Read the model definition and answer for the solid it produces. Units are mm, in the model's axes. Face numbers are marked on the shaded views. A direction names the side the tool comes from. Give positions to 0.01 mm unless a question says otherwise; leave off trailing zeros. Write each loop counter-clockwise with the first axis right and the second up, starting at its lowest first coordinate (ties: lowest second). Pieces come first, ordered by that corner, then holes. Notation, with made-up numbers: M 35.25,58 L 78.25,58 A11 cw 78.25,63 Z; hole C 68.5,-32 d7. An arc over 180 degrees is marked long. Answer as CSV lines item,"result". Start each with the question number.
Autodesk Inventor part; units mm, degrees
ref_plane "Work Plane1" through (29, 0, 0) normal (0, -1, 0) x (1, 0, 0)
ref_plane "YZ Plane" through (0, 0, 0) normal (1, 0, 0) x (0, 1, 0)
ref_plane "XZ Plane" through (0, 0, 0) normal (0, 1, 0) x (-1, 0, 0)
sketch "Sketch1" plane through (0, 0, 0) normal (0, 0, 1) x (1, 0, 0)
  line L0 (-1.1667, 0) -> (35, 0)
  line L1 (35, 0) -> (35, 2.5)
  line L2 (35, 2.5) -> (19, 2.5)
  line L3 (19, 2.5) -> (18.5091, 2.5)
  line L4 (18.5091, 2.5) -> (0, 2.5)
  line L5 (0, 2.5) -> (0, 4.25)
  line L6 (0, 4.25) -> (-5, 4.25)
  line L7 (-5, 4.25) -> (-5, 2.3094)
  line L8 (-5, 2.3094) -> (-2.5, 2.3094)
  line L9 (-2.5, 2.3094) -> (-1.1667, 0)
  line L10 (-13, 0) -> (43, 0)
  line L11 (0, -0.85) -> (0, 5.1)
  line L12 (19, 2.5) -> (0, 2.5) construction
  dimension "d1" = 16
  dimension "d2" = 0.4909
  dimension "d3" = 5
  dimension "d4" = 2.5
  dimension "d5" = 60
  dimension "d6" = 5
  dimension "d7" = 5
  dimension "d8" = 4.6188
  dimension "d9" = 8.5
  dimension "d26" = 35
revolve "Body" add sketch "Sketch1" angle 360 about axis through (-1.1667, 0, 0) along (1, 0, 0)
sketch "Sketch2" plane through (-5, 0, 0) normal (-1, 0, 0) x (0, 0, 1)
  circle A0 centre (0, 0) radius 2.3094
  line L0 (0, -5.95) -> (0, 5.95)
  line L1 (-5.95, 0) -> (5.95, 0)
  line L2 (2.3094, 0) -> (1.1547, -2)
  line L3 (1.1547, -2) -> (-1.1547, -2)
  line L4 (-1.1547, -2) -> (-2.3094, 0)
  line L5 (-2.3094, 0) -> (-1.1547, 2)
  line L6 (-1.1547, 2) -> (1.1547, 2)
  line L7 (1.1547, 2) -> (2.3094, 0)
extrude "Slot" add sketch "Sketch2" against normal up to next contours L7 A0 | A0 L2 | L6 L0 A0 | A0 L0 L3 | L0 L6 A0 | A0 L3 L0 | L4 A0 | A0 L5
fillet "Fillet1" radius 0.5 1 edges at (-5, -4.25, 0)
thread "Thread"
chamfer "Chamfer1" distance 0.4908 distance2 0.4908 1 edges at (35, -2.5, 0) measured on face at (35, -0.7192, 0.1653)
ref_plane "Work Plane1" through (29, 0, 0) normal (0, -1, 0) x (1, 0, 0)
fillet "Fillet2" radius 0.1 1 edges at (0, -2.5, 0)
equation "\"d1\" = GEL"
equation "\"d3\" = KOH"
equation "\"d4\" = INTI"
equation "\"d6\" = GD"
equation "\"d7\" = BDM"
equation "\"d8\" = 1.1547 * SW"
equation "\"d9\" = KOD"
equation "\"d17\" = RR"
equation "\"d13\" = GEL"
equation "\"d15\" = -0.5 * SPD + 0.5 * GD"
equation "\"d16\" = GUL"
equation "\"d30\" = R"
equation "\"GD\" = NND"
equation "\"GEL\" = 16"
equation "\"KOD\" = 8.5"
equation "\"KOH\" = NND"
equation "\"INTI\" = 2.5"
equation "\"GAL\" = 0.61345 * PTC"
equation "\"GUL\" = 0.61345 * PTC"
equation "\"BDM\" = NND"
equation "\"SW\" = 4"
equation "\"RR\" = 0.1 * NND"
equation "\"SPD\" = NND - 1.2269 * PTC"
equation "\"R\" = 0.1"
equation "\"PHH\" = 0.13"
equation "\"GD1\" = THREADDIA - 1.2269 * PTC"
equation "\"THREADDIA\" = 5"
equation "\"FAWI\" = 45deg"
equation "\"PTC\" = 0.8"
equation "\"KOH1\" = 4.5"
equation "\"NND\" = 5"
equation "\"TOA\" = 30deg"
equation "\"E0\" = 1.155 * SW"
properties part number "AS 1420 - 1973 - M5 x 20" material "Steel, Mild"
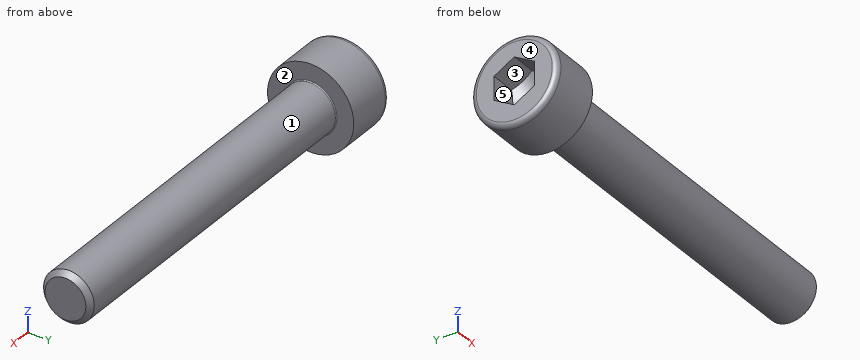
1. Find section A-A on x = 14. Determine the outline of the cut face in (y, z).
2. Determine the mould class of the marked faces 1, 2 and 3 for opening direction Y: +Y half, -Y half, draft (parallel to the pull), parting line (faces both ways), or undercut.
3. Find the intervals of material crossed by line 1 (Z direction, x = 25.5, y = -1.5); line 2 (X direction, y = -2.5, z = 1.25), in increasing order. Write a range as [from, to].
4. Given pin 1 (5 mm diameter, centred on x = 11, y = -3.5, fed in from +Z); pin 2 (1.5 mm diameter, centred on x = 7.5, y = 1.5, fed in from -Z); pin 3 (1.5 mm diameter, centred on y = -3, z = 3.5, fed in from -X), each flat-ended and moving along its own axis, determine where each tip first touches the part or whether it passes through.
5. For the marked faces 4 and 5, determine the directions among +Z, -Z, +X, -X, +Y, -Y from which every point of the face is accessible in a straight line to the end or side of a thin tool.
Computed:
1,outline,"C 0,0 d5"
2,face 1,"parting line"
2,face 2,"draft"
2,face 3,"undercut"
3,line 1,"z = [-2, 2]"
3,line 2,"x = [-5, 0]"
4,pin 1,"stops at z = 2.29"
4,pin 2,"stops at z = -2.38"
4,pin 3,"stops at x = -4.99"
5,face 4,"+Z, -Z, -X, +Y, -Y"
5,face 5,"-X"
